Geometry: final body of the model. Coordinates: model frame, mm. Face numbers are marked on the shaded views. Give positions to 0.01 mm unless a question says otherwise; leave off trailing zeros. Write each loop counter-clockwise with the first axis right and the second up, starting at its lowest first coordinate (ties: lowest second). Pieces come first, ordered by that corner, then holes. Notation, with made-up numbers: (-32, 14.25) -> (26, 14.25) arc R6 cw to (26, 21.25) -> close; hole circle Ø5 at (22, 83.25). An arc over 180 degrees is marked (long way). Answer in a Markdown table with one row per item. Add a question column.
Item 1: Draft query along Y for the marked faces 1 and 2. Return one class per face: +Y half, -Y half, draft (parallel to the pull), parting line (faces both ways), or undercut.
Item 2: Section query B-B on z = -282. Output: boundary loops of the cut face in (x, y), plus the area to 3 significant figures.
Item 3: Material intervals for probe 1 along Y at (x, z) = (294, -461); probe 2 along Z at (x, y) = (302.5, 224); probe 3 along X at (y, z) = (16, -268), sorted ascending. Write a range as from..to.
Item 4: Section query A-A on y = 174. Output: boundary loops of the cut face in (x, z), plus the area to 3 significant figures.
```python
from build123d import *

# Parameters (mm, degrees)
F3_R = 20


with BuildPart() as f4:
    # F4: sweep along a path in F0, F2
    with BuildLine(Plane.XZ) as f4_path:
        Line((0, 0), (100, 0))
        ThreePointArc((100, 0), (241.4213562373, -58.5786437627), (300, -200))
    with BuildLine(Plane.YZ.offset(300)) as f4_path_2:
        Line((0, -200), (0, -450))
        ThreePointArc((0, -450), (43.933982822, -556.066017178), (150, -600))
        Line((150, -600), (250, -600))
        ThreePointArc((250, -600), (356.066017178, -556.066017178), (400, -450))
        Line((400, -450), (400, -400))
    # F3 (on Right) → F4 (sweep)
    with BuildSketch(Plane.YZ):
        Circle(F3_R)
    sweep(path=f4_path.line + f4_path_2.line)


solid = f4.part
```
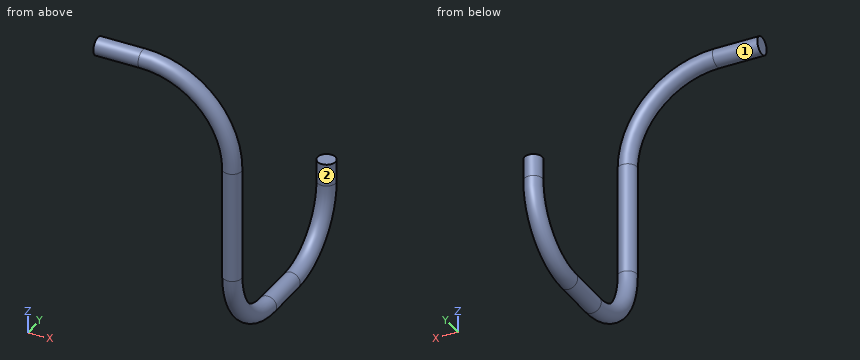
Findings below:
| question | item | result |
|---|---|---|
| 1 | face 1 | parting line |
| 1 | face 2 | undercut |
| 2 | outline | circle Ø40 at (300, 0) |
| 2 | area | 1,260 mm^2 |
| 3 | probe 1 | y = -18.72..19.54, 380.46..418.72 |
| 3 | probe 2 | z = -619.84..-580.16 |
| 3 | probe 3 | x = 288..312 |
| 4 | outline | circle Ø40 at (300, -600) |
| 4 | area | 1,260 mm^2 |
